For this review, take the finished solid that the model builds, in its own axes (mm). Round coordinates to 2 decimals unless told otherwise and drop trailing zeros. Write each loop counter-clockwise with the first axis right and the second up, starting at its lowest first coordinate (ties: lowest second). Pieces come first, ordered by that corner, then holes. Notation, with made-up numbers: M 34.5,4.25 L 68.5,4.25 A17 ccw 68.5,20.25 Z; hole C 0.5,78 d8. An arc over 180 degrees is marked long. Write each question's results on one line, items separated by ' | '. Start each with the question number.
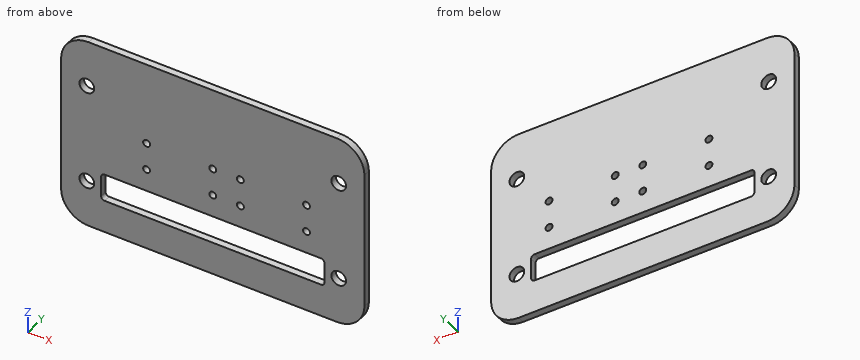
```python
from build123d import *

# Parameters (mm, degrees)
SKETCH3_W                   = 69.85
SKETCH3_H                   = 44.45
BOSS_EXTRUDE1_DEPTH         = 1.5875
M3_CLEARANCE_HOLE1_D        = 3.4
TAP_DRILL_FOR_M2X0_4_TAP1_D = 1.6
FILLET1_R                   = 6.35
SKETCH8_W                   = 51.425
SKETCH8_H                   = 6.35
CUT_EXTRUDE1_DEPTH          = 2.5875
FILLET2_R                   = 0.79375


with BuildPart() as part:
    # Sketch3 → Boss-Extrude1 (new body)
    with BuildSketch(Plane(origin=(0, 0, 0), x_dir=(1, 0, 0), z_dir=(0, 1, 0))):
        Rectangle(SKETCH3_W, SKETCH3_H)
    extrude(amount=BOSS_EXTRUDE1_DEPTH)

    # M3 Clearance Hole1 (through all)
    with Locations(Plane(origin=(0, 1.5875, 0), x_dir=(1, 0, 0), z_dir=(0, 1, 0))):
        with Locations((-29, 11.5), (-29, -11.5), (29, -11.5), (29, 11.5)):
            Hole(M3_CLEARANCE_HOLE1_D / 2)

    # Tap Drill for M2x0.4 Tap1 (through all)
    with Locations(Plane(origin=(0, 1.5875, 0), x_dir=(1, 0, 0), z_dir=(0, 1, 0))):
        with Locations((21.59, -3.175), (-15.24, 3.175), (0, 3.175), (-15.24, -3.175), (0, -3.175), (6.35, 3.175), (21.59, 3.175), (6.35, -3.175)):
            Hole(TAP_DRILL_FOR_M2X0_4_TAP1_D / 2)

    # Fillet1
    fillet1_edges = [part.edges().sort_by_distance(p)[0] for p in [
        (34.925, 0.79375, 22.225),
        (-34.925, 0.79375, 22.225),
        (-34.925, 0.79375, -22.225),
        (34.925, 0.79375, -22.225),
    ]]
    fillet(fillet1_edges, radius=FILLET1_R)

    # Sketch8 → Cut-Extrude1 (cut, through all)
    with BuildSketch(Plane(origin=(0, 1.5875, 0), x_dir=(1, 0, 0), z_dir=(0, 1, 0))):
        with Locations((0, 11.5)):
            Rectangle(SKETCH8_W, SKETCH8_H)
    extrude(amount=-CUT_EXTRUDE1_DEPTH, mode=Mode.SUBTRACT)

    # Fillet2
    fillet2_edges = [part.edges().sort_by_distance(p)[0] for p in [
        (-25.7125, 0.79375, -8.325),
        (-25.7125, 0.79375, -14.675),
        (25.7125, 0.79375, -14.675),
        (25.7125, 0.79375, -8.325),
    ]]
    fillet(fillet2_edges, radius=FILLET2_R)


solid = part.part
```
Item 1: We need section A-A on z = -11.5. State the section outline as (x, y) points (1 decimal), then the cut area to 3 significant figures.
Item 2: We need section D-D on x = -29.5. State the section outline as (y, z) points, then the cut area to 3 significant figures.
Item 3: Insertion check: P1, Ø1.4, axis at x = 6.35, z = 3.175, coming from the +Y side. The pin has a flat end and moves straight along its axis. Give the tip position at first contact, or say it passes through.
Item 4: We need section C-C on y = 0.5. State how many separate pieces and enclosed holes the cut face has, then the cut area to 3 significant figures.
Item 5: We need section B-B on x = 6.35. State the section outline as (y, z) points (1 decimal), then the cut area to 3 significant figures.
Item 6: For probe 1 along Z at (x, y) = (-15.24, 0.4) (3 decimals); probe 2 along Z at (x, y) = (29, 1.15); probe 3 along X at (y, z) = (1.05, 11.5) (3 decimals), list the stretches that pass through material, from the lowest coordinate up.
Numbers:
1) outline: M -34.9,0 L -30.7,0 L -30.7,1.6 L -34.9,1.6 Z; M -27.3,0 L -25.7,0 L -25.7,1.6 L -27.3,1.6 Z; M 25.7,0 L 27.3,0 L 27.3,1.6 L 25.7,1.6 Z; M 30.7,0 L 34.9,0 L 34.9,1.6 L 30.7,1.6 Z | area: 18.5 mm^2
2) outline: M 0,-22.16 L 1.59,-22.16 L 1.59,-13.12 L 0,-13.12 Z; M 0,-9.88 L 1.59,-9.88 L 1.59,9.88 L 0,9.88 Z; M 0,13.12 L 1.59,13.12 L 1.59,22.16 L 0,22.16 Z | area: 60.0 mm^2
3) P1: passes through
4) separate pieces: 1 | enclosed holes: 13 | area: 2,690 mm^2
5) outline: M 0,-22.2 L 1.6,-22.2 L 1.6,-14.7 L 0,-14.7 Z; M 0,-8.3 L 1.6,-8.3 L 1.6,-4 L 0,-4 Z; M 0,-2.4 L 1.6,-2.4 L 1.6,2.4 L 0,2.4 Z; M 0,4 L 1.6,4 L 1.6,22.2 L 0,22.2 Z | area: 55.4 mm^2
6) probe 1: z = -22.225 to -14.675, -8.325 to -3.975, -2.375 to 2.375, 3.975 to 22.225 | probe 2: z = -22.21 to -13.2, -9.8 to 9.8, 13.2 to 22.21 | probe 3: x = -34.925 to -30.7, -27.3 to 27.3, 30.7 to 34.925
